Model file for the job. Use its own axes, mm. A direction names the side the tool comes from. Coordinates: 2 decimals unless noted, no trailing zeros. Order: outer loops, then holes, each group sorted by start corner. A loop starts at its lowest first (then second) coordinate and runs counter-clockwise, first axis right, second up. Notation, with made-up numbers: M -3,-4.75 L 3,-4.75 A20 cw 3,8.25 Z; hole C 77,86 d3. An arc over 180 degrees is marked long. Return JSON: item names as keys, results as strings.
```python
from build123d import *

# Parameters (mm, degrees)
SKETCH1_W           = 35.76
SKETCH1_H           = 90
BOSS_EXTRUDE1_DEPTH = 15
SKETCH2_W           = 53.76
SKETCH2_H           = 108
BOSS_EXTRUDE2_DEPTH = 2.5
SHELL1_START        = -15.38
SHELL1_OUTLINE_W    = 85
SHELL1_OUTLINE_H    = 15
SHELL1_DEPTH        = 30.76
FILLET1_R           = 2.5
FILLET2_R           = 5
SKETCH3_W           = 15
SKETCH3_H           = 8
CUT_EXTRUDE1_DEPTH  = 63.15733585
SKETCH4_R           = 1.25
CUT_EXTRUDE2_DEPTH  = 2.5


# Read off the part's stored shape, not the designer's step: Shell1
with BuildPart() as part:
    # Sketch1 → Boss-Extrude1 (new body)
    with BuildSketch(Plane.XY):
        Rectangle(SKETCH1_W, SKETCH1_H)
    extrude(amount=BOSS_EXTRUDE1_DEPTH)

    # Sketch2 → Boss-Extrude2 (add)
    with BuildSketch(Plane.XY.offset(15)):
        Rectangle(SKETCH2_W, SKETCH2_H)
    extrude(amount=BOSS_EXTRUDE2_DEPTH)

    # Shell1 outline → Shell1 (cut)
    with BuildSketch(Plane.YZ.offset(SHELL1_START)):
        with Locations((0, 10)):
            Rectangle(SHELL1_OUTLINE_W, SHELL1_OUTLINE_H)
    extrude(amount=SHELL1_DEPTH, mode=Mode.SUBTRACT)

    # Fillet1
    fillet1_edges = [part.edges().sort_by_distance(p)[0] for p in [
        (26.88, -54, 16.25),
        (26.88, 54, 16.25),
        (-26.88, 54, 16.25),
        (-26.88, -54, 16.25),
    ]]
    fillet(fillet1_edges, radius=FILLET1_R)

    # Fillet2
    fillet2_edges = [part.edges().sort_by_distance(p)[0] for p in [
        (15.38, 0, 2.5),
        (0, 42.5, 2.5),
        (-15.38, 0, 2.5),
        (0, -42.5, 2.5),
        (0, -45, 0),
        (-17.88, 0, 0),
        (0, 45, 0),
        (17.88, 0, 0),
    ]]
    fillet(fillet2_edges, radius=FILLET2_R)

    # Sketch3 → Cut-Extrude1 (cut, through all)
    with BuildSketch(Plane.XY.offset(2.5)):
        with Locations((0, 25)):
            Rectangle(SKETCH3_W, SKETCH3_H)
    extrude(amount=-CUT_EXTRUDE1_DEPTH, mode=Mode.SUBTRACT)

    # Sketch4 → Cut-Extrude2 (cut)
    with BuildSketch(Plane.XY.offset(17.5)):
        with Locations((-22.63, 49.5)):
            Circle(SKETCH4_R)
        with Locations((22.63, 49.5)):
            Circle(SKETCH4_R)
        with Locations((22.63, 24.75)):
            Circle(SKETCH4_R)
        with Locations((22.63, 0)):
            Circle(SKETCH4_R)
        with Locations((22.63, -24.75)):
            Circle(SKETCH4_R)
        with Locations((22.63, -49.5)):
            Circle(SKETCH4_R)
        with Locations((-22.63, 24.75)):
            Circle(SKETCH4_R)
        with Locations((-22.63, 0)):
            Circle(SKETCH4_R)
        with Locations((-22.63, -24.75)):
            Circle(SKETCH4_R)
        with Locations((-22.63, -49.5)):
            Circle(SKETCH4_R)
    extrude(amount=-CUT_EXTRUDE2_DEPTH, mode=Mode.SUBTRACT)


solid = part.part
```
Item 1: Saw through at A-A (y = 24.75). Write the cut outline in (x, z), and give its area (3 significant figures).
Check result:
{"outline": "M -26.88,15 L -23.88,15 L -23.88,17.5 L -26.88,17.5 Z; M -21.38,15 L -17.88,15 L -17.88,5 A5 ccw -12.88,0 L -7.5,0 L -7.5,2.5 L -10.38,2.5 A5 cw -15.38,7.5 L -15.38,17.5 L -21.38,17.5 Z; M 7.5,0 L 12.88,0 A5 ccw 17.88,5 L 17.88,15 L 21.38,15 L 21.38,17.5 L 15.38,17.5 L 15.38,7.5 A5 cw 10.38,2.5 L 7.5,2.5 Z; M 23.88,15 L 26.88,15 L 26.88,17.5 L 23.88,17.5 Z", "area": "159 mm2"}
Item 2: Wall check: line 1 (Y direction, x = -22.63, z = 17.05); line 2 (X direction, y = 36.5, z = 14.5); line 3 (X direction, y = 8.5, z = 15.5). Give the ranges that are in metal, low to high.
Check result:
{"line 1": "y = -54 to -50.75, -48.25 to -26, -23.5 to -1.25, 1.25 to 23.5, 26 to 48.25, 50.75 to 54", "line 2": "x = -17.88 to -15.38, 15.38 to 17.88", "line 3": "x = -26.88 to -15.38, 15.38 to 26.88"}
Item 3: Saw through at C-C (z = 11). Write the cut outline in (x, y).
Check result:
{"outline": "M -17.88,-45 L 17.88,-45 L 17.88,45 L -17.88,45 Z; hole M -15.38,-42.5 L 15.38,-42.5 L 15.38,42.5 L -15.38,42.5 Z"}
Item 4: Drop flat-ended pins along their axis: pin 1 Ø5 at (x, z) = (4.5, 6) entering from -Y; pin 2 Ø1.2 at (x, z) = (-1, 1) entering from +Y; pin 3 Ø3 at (x, z) = (1.5, 10.5) entering from +Y; pin 4 Ø2 at (x, y) = (22.63, -24.75) entering from +Z. Give the stop position or say it passes through.
Check result:
{"pin 1": "stops at y = -45", "pin 2": "stops at y = 43.67", "pin 3": "stops at y = 45", "pin 4": "passes through"}
Item 5: 3-axis set-ups, long thin cutter, end or side, ignore diameter. For faces 1 (the flat face through (0, -45, 10)), 2 (the flat face through (0, 29, 1)), 3 (the cylindrical face through (0.22, -41.07, 4)): which of +Z, -Z, +X, -X, +Y, -Y reach the whole face in a straight line?
Check result:
{"face 1": "-Z, +X, -X, -Y", "face 2": "+Z, -Z", "face 3": "+Z"}
Item 6: Saw through at B-B (x = -22.63). Write the cut outline in (y, z).
Check result:
{"outline": "M -54,15 L -50.75,15 L -50.75,17.5 L -54,17.5 Z; M -48.25,15 L -26,15 L -26,17.5 L -48.25,17.5 Z; M -23.5,15 L -1.25,15 L -1.25,17.5 L -23.5,17.5 Z; M 1.25,15 L 23.5,15 L 23.5,17.5 L 1.25,17.5 Z; M 26,15 L 48.25,15 L 48.25,17.5 L 26,17.5 Z; M 50.75,15 L 54,15 L 54,17.5 L 50.75,17.5 Z"}
Item 7: Saw through at D-D (y = -24.75). Write the cut outline in (x, z).
Check result:
{"outline": "M -26.88,15 L -23.88,15 L -23.88,17.5 L -26.88,17.5 Z; M -21.38,15 L -17.88,15 L -17.88,5 A5 ccw -12.88,0 L 12.88,0 A5 ccw 17.88,5 L 17.88,15 L 21.38,15 L 21.38,17.5 L 15.38,17.5 L 15.38,7.5 A5 cw 10.38,2.5 L -10.38,2.5 A5 cw -15.38,7.5 L -15.38,17.5 L -21.38,17.5 Z; M 23.88,15 L 26.88,15 L 26.88,17.5 L 23.88,17.5 Z"}
Item 8: Pull direction Y, two halves, no side cores. Call faces 4 (the cylindrical face through (-23.551, 50.345, 16.267)), 5 (the cylindrical face through (0, 44, 2)), 6 (the flat face through (-18, 1, 17.5)), 7 (the cylindrical face through (-26.167, -53.248, 16.267)): +Y half, -Y half, draft (parallel to the pull), parting line (faces both ways), or undercut.
Check result:
{"face 4": "undercut", "face 5": "+Y half", "face 6": "draft", "face 7": "-Y half"}
